Check sheet for the modelled part. Datum: model origin and axes. Units: mm. A direction names the side the tool comes from. Coordinates: 2 decimals unless noted, no trailing zeros. Write each loop counter-clockwise with the first axis right and the second up, starting at its lowest first coordinate (ties: lowest second). Pieces come first, ordered by that corner, then holes. Notation, with made-up numbers: (-7, -11) -> (31, -11) arc R26 ccw to (31, 11) -> close; hole circle Ø8 at (-36, 59.5). An arc over 180 degrees is marked (long way). One line per item, written item: value. Start each with the question number.
1) Set-up check for faces 4 (the flat face through (-31.75, 35, 86)), 5 (the flat face through (0, 1, 20)), 6 (the flat face through (-35, -38.1, 86)), 7 (the flat face through (-35, -31.75, 86)), 8 (the flat face through (35, 38.1, 86)): record each of +Z, -Z, +X, -X, +Y, -Y from which the full face is reachable in a straight line by a thin tool's end or side.
2) Scan lines: line 1 along Z through (x, y) = (-29, 10); line 2 along Z through (x, y) = (-21.5, -27); line 3 along X through (y, z) = (12, 62). Record each from-to range of solid material in increasing order. Write a range as [from, to].
3) Gauge pin test, flat ends, axial feed: P1, Ø1.5, axis at y = 3.5, z = 27, coming from the +X side; P2, Ø5, axis at x = 32, z = 127.5, coming from the +Y side; P3, Ø7, axis at y = 35, z = 79.5, coming from the -X side. Record the tip position at first contact, or that the pin passes through.
4) Sectioned sample at A-A on z = 32.5. Enter the section's corners in (x, y), plus the area to 3 significant figures.
5) Draft check along Z on faces 1 (the flat face through (24, 1, 0)), 2 (the flat face through (54.33, 22.14, 20.04)), 3 (the flat face through (1, -1, 71.12)). Enter one of: +Z half, -Z half, draft (parallel to the pull), parting line (faces both ways), or undercut.
```python
from build123d import *

# Parameters (mm, degrees)
F2_DEPTH = 40.64
F7_W     = 6.35
F7_H     = 6.35
F8_DEPTH = 30.48


with BuildPart() as f2:
    # F1 (on Top) → F2 (new body)
    with BuildSketch(Plane.XY):
        Polygon((44.901281, 44.901281), (0, 63.5), (0, -63.5), (44.901281, -44.901281), (63.5, 0), align=None)
    extrude(amount=F2_DEPTH)

    # F3 (on offset) → F6 section 0
    with BuildSketch(Plane.XY.offset(40.64)):
        Polygon((0, -63.5), (44.901281, -44.901281), (63.5, 0), (44.901281, 44.901281), (0, 63.5), (-44.901281, 44.901281), (-63.5, 0), (-44.901281, -44.901281), align=None)
    # F5 (on offset) → F6 section 1
    with BuildSketch(Plane.XY.offset(71.12)):
        Polygon((0, 53.881537), (-38.1, 38.1), (-53.881537, 0), (-38.1, -38.1), (0, -53.881537), (38.1, -38.1), (53.881537, 0), (38.1, 38.1), align=None)
    loft()

    # F7 (on offset) → F8 (join)
    with BuildSketch(Plane.XY.offset(71.12)):
        with Locations((-34.925, 34.925)):
            Rectangle(F7_W, F7_H)
        with Locations((34.925, 34.925)):
            Rectangle(F7_W, F7_H)
        with Locations((34.925, -34.925)):
            Rectangle(F7_W, F7_H)
        with Locations((-34.925, -34.925)):
            Rectangle(F7_W, F7_H)
    extrude(amount=F8_DEPTH)

    # F12 (on Front) → F13 (revolve)
    with BuildSketch(Plane.XZ):
        with BuildLine():
            ThreePointArc((0, 146.05), (-36.511636, 134.029246), (-57.15, 101.6))
            Line((-57.15, 101.6), (0, 101.6))
            Line((0, 101.6), (0, 146.05))
        make_face()
    revolve(axis=Axis((0, 0, 123.825), (0, 0, 1)))


solid = f2.part
```
Answers:
1. face 4: +Y, -Y
1. face 5: -Z, -X, +Y, -Y
1. face 6: +X, -X, -Y
1. face 7: +X, -X
1. face 8: +X, -X, +Y
2. line 1: z = [40.64, 71.12], [101.6, 138.01]
2. line 2: z = [40.64, 71.12], [101.6, 135.51]
2. line 3: x = [-51.79, 51.79]
3. P1: stops at x = 62.36
3. P2: stops at y = 33.54
3. P3: stops at x = -38.1
4. outline: (0, -63.5) -> (44.9, -44.9) -> (63.5, 0) -> (44.9, 44.9) -> (0, 63.5) -> close
4. area: 5,700 mm2
5. face 1: -Z half
5. face 2: draft
5. face 3: undercut
